Source: three-view drawing plus pictorial views. Frame: mm from the lowest corner of the part. Give positions to 0.01 mm unless a question says otherwise; leave off trailing zeros. Loops run counter-clockwise (first coordinate to the right, second up) from the corner with the lowest first, then second, coordinate; pieces in that order, holes last.
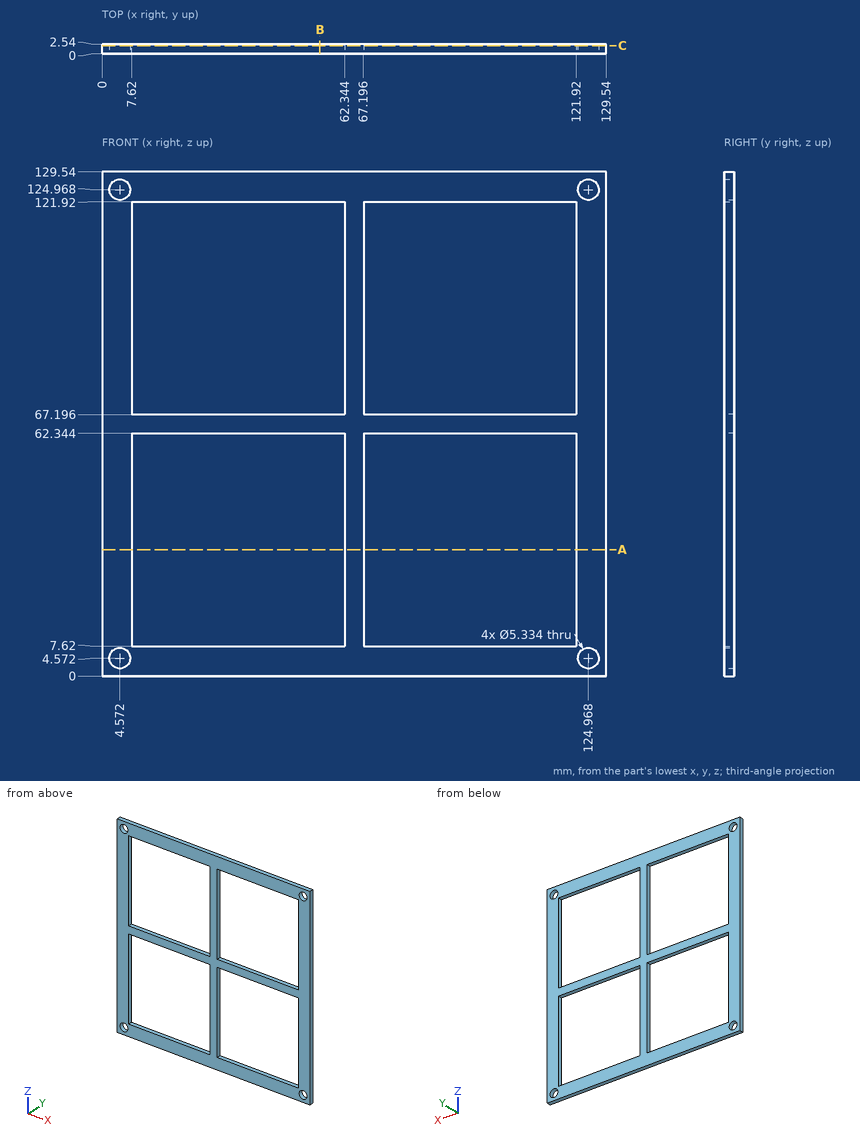
(1) Ray query, probe 1 along X at (y, z) = (2, 110); probe 2 along Z at (x, y) = (7, 0.75) (1 decimal). Return the intervals inside material, ascending.
Values follow:
probe 1: x = 0 to 7.62, 62.34 to 67.2, 121.92 to 129.54
probe 2: z = 0 to 3.5, 5.7 to 123.9, 126.1 to 129.5
(2) Pin query (flat end, axial travel): pin 1 Ø5 at (x, z) = (4.572, 4.572) entering from -Y. Return the tip coordinate at first contact, or that it passes through.
Values follow:
pin 1: passes through
(3) Cut plane C-C (y = 2.15). Count the separate pieces of the cut face and the enclosed holes in it, and give its area (3 significant figures).
Values follow:
separate pieces: 1
enclosed holes: 8
area: 4,710 mm2
(4) Cut plane B-B (x = 56). Return the cut outline in (y, z).
Values follow:
outline: (0, 0) - (2.54, 0) - (2.54, 7.62) - (0, 7.62) - close; (0, 62.34) - (2.54, 62.34) - (2.54, 67.2) - (0, 67.2) - close; (0, 121.92) - (2.54, 121.92) - (2.54, 129.54) - (0, 129.54) - close
(5) Cut plane A-A (z = 32.5). Return the cut outline in (x, y).
Values follow:
outline: (0, 0) - (7.62, 0) - (7.62, 2.54) - (0, 2.54) - close; (62.34, 0) - (67.2, 0) - (67.2, 2.54) - (62.34, 2.54) - close; (121.92, 0) - (129.54, 0) - (129.54, 2.54) - (121.92, 2.54) - close
